Geometry: final body of the model. Coordinates: model frame, mm. A direction names the side the tool comes from. Round coordinates to 2 decimals unless told otherwise and drop trailing zeros. Loops run counter-clockwise (first coordinate to the right, second up) from the corner with the lowest first, then second, coordinate; pieces in that order, holes last. Notation, with made-up numbers: (18, 45.25) - (41, 45.25) arc R16 cw to (41, 52.25) - close; hole circle Ø4 at (51.5, 63). An arc over 180 degrees is marked (long way). Return JSON: item names as keys, results as strings. Group by question number.
1. Set-up query: faces 4 (the face through (8.159, 15.605, 22.715)), 5 (the face through (-22.3, -1, 23)), 6 (the face through (-13.529, -0.685, -18.532)). Return all of +Z, -Z, +X, -X, +Y, -Y with unobstructed straight access to the full face (end or side cutting, diameter ignored); none if empty.
2. Draft query along Z for faces 1 (the face through (-16, -1, 20.25)), 2 (the face through (-20.87, 47.4, 22.72)), 3 (the face through (0, -1, 25.25)). Return one class per face: +Z half, -Z half, draft (parallel to the pull), parting line (faces both ways), or undercut.
3. Section D-D on x = 15.5. Return loops of the section in (y, z).
4. Material intervals for probe 1 along Y at (x, z) = (-11.25, 23.15); probe 2 along Z at (x, y) = (0.5, -32.4); probe 3 along X at (y, z) = (3.5, -10), sorted ascending.
5. Section C-C on y = 24. Return loops of the section in (x, z), and give its area (3 significant figures).
6. Section A-A on x = 4. Return loops of the section in (y, z), and give its area (3 significant figures).
7. First-contact query: pin 1 Ø10.5 at (x, y) = (-11.25, 10.76) entering from +Z; pin 2 Ø9.5 at (y, z) = (-11, 10.5) entering from +X; pin 3 Ø9.5 at (y, z) = (-5.5, 9) entering from -X. Flat tips, straight axial feed; report the tip coordinate or a pass-through.
8. Section B-B on z = 0. Return loops of the section in (x, y), and give its area (3 significant figures).
from build123d import *

# Parameters (mm, degrees)
F1_DEPTH = 48.9
F3_R     = 5
F5_D     = 11
F7_D     = 11.5
F7_DEPTH = 12
F7_TIP   = 3.4549485594


# Not quite as in the source:
# - a feature names something its author has since deleted; it is built from what else it names


with BuildPart() as f1:
    # F0 (on Front) → F1 (new body, symmetric)
    with BuildSketch(Plane.XZ):
        Polygon((-5, 20.25), (5, 20.25), (22.3, 20.25), (22.3, 25.25), (-22.3, 25.25), (-22.3, 20.25), align=None)
        Polygon((5, 0), (5, 20.25), (-5, 20.25), (-5, -12), (-5, -20.25), (0, -20.25), (5, -20.25), (5, -12), align=None)
        Polygon((-5, -20.25), (-5, -12), (-22.3, -25.25), (-22.3, -30.25), (22.3, -30.25), (22.3, -25.25), (5, -12), (5, -20.25), (0, -20.25), align=None)
    extrude(amount=F1_DEPTH, both=True)

    # F3
    f3_edges = [f1.edges().sort_by_distance(p)[0] for p in [
        (-22.3, 48.9, 22.75),
        (-22.3, -48.9, 22.75),
        (22.3, 48.9, 22.75),
        (22.3, -48.9, 22.75),
        (-22.3, -48.9, -27.75),
        (22.3, -48.9, -27.75),
        (-22.3, 48.9, -27.75),
        (22.3, 48.9, -27.75),
    ]]
    fillet(f3_edges, radius=F3_R)

    # F5 (through all)
    with Locations(Plane(origin=(-5, 0, 0), x_dir=(0, -1, 0), z_dir=(-1, 0, 0))):
        with Locations((32.4, 0), (10.8, 0), (-10.8, 0), (-32.4, 0)):
            Hole(F5_D / 2)

    # F7
    with Locations(Plane.XY.offset(25.25)):
        with Locations((-11.25, 32.5910784304), (11.25, 32.5910784304), (11.25, 10.7566630468), (-11.25, 10.7566630468), (-11.25, -10.7566630468), (11.25, -10.7566630468), (11.25, -32.5910784304), (-11.25, -32.5910784304)):
            Hole(F7_D / 2, depth=F7_DEPTH)
            with Locations((0, 0, -(F7_DEPTH + F7_TIP / 2))):  # 118° drill point
                Cone(0, F7_D / 2, F7_TIP, mode=Mode.SUBTRACT)


solid = f1.part
Taken from the geometry:
{
 "1": {"face 4": "+Z", "face 5": "+Z, -Z, -X, +Y, -Y", "face 6": "-X, +Y, -Y"},
 "2": {"face 1": "undercut", "face 2": "draft", "face 3": "+Z half"},
 "3": {"outline": "(-48.9, -30.25) - (48.9, -30.25) - (48.9, -20.04) - (-48.9, -20.04) - close; (-48.9, 20.25) - (-36.46, 20.25) - (-36.46, 25.25) - (-48.9, 25.25) - close; (-28.72, 20.25) - (-14.63, 20.25) - (-14.63, 25.25) - (-28.72, 25.25) - close; (-6.88, 20.25) - (6.88, 20.25) - (6.88, 25.25) - (-6.88, 25.25) - close; (14.63, 20.25) - (28.72, 20.25) - (28.72, 25.25) - (14.63, 25.25) - close; (36.46, 20.25) - (48.9, 20.25) - (48.9, 25.25) - (36.46, 25.25) - close"},
 "4": {"probe 1": "-48.9 to -38.34, -26.84 to -16.51, -5.01 to 5.01, 16.51 to 26.84, 38.34 to 48.9", "probe 2": "-30.25 to -5.5, 5.5 to 25.25", "probe 3": "-5 to 5"},
 "5": {"outline": "(-22.3, -30.25) - (22.3, -30.25) - (22.3, -25.25) - (5, -12) - (5, 20.25) - (22.3, 20.25) - (22.3, 25.25) - (-22.3, 25.25) - (-22.3, 20.25) - (-5, 20.25) - (-5, -12) - (-22.3, -25.25) - close", "area": "1,130 mm2"},
 "6": {"outline": "(-48.9, -30.25) - (48.9, -30.25) - (48.9, 25.25) - (-48.9, 25.25) - close; hole circle Ø11 at (-32.4, 0); hole circle Ø11 at (-10.8, 0); hole circle Ø11 at (10.8, 0); hole circle Ø11 at (32.4, 0)", "area": "5,050 mm2"},
 "7": {"pin 1": "z = -12.77", "pin 2": "x = 5", "pin 3": "x = -5"},
 "8": {"outline": "(-5, -48.9) - (5, -48.9) - (5, -37.9) - (-5, -37.9) - close; (-5, -26.9) - (5, -26.9) - (5, -16.3) - (-5, -16.3) - close; (-5, -5.3) - (5, -5.3) - (5, 5.3) - (-5, 5.3) - close; (-5, 16.3) - (5, 16.3) - (5, 26.9) - (-5, 26.9) - close; (-5, 37.9) - (5, 37.9) - (5, 48.9) - (-5, 48.9) - close", "area": "538 mm2"}
}
